Work out the finished part from the listing and answer in its coordinate system (mm). Round coordinates to 2 decimals unless told otherwise and drop trailing zeros. Write each loop counter-clockwise with the first axis right and the second up, starting at its lowest first coordinate (ties: lowest second). Pieces come first, ordered by that corner, then holes. Notation, with made-up numbers: M -7.5,55.25 L 7.5,55.25 A20 ccw 7.5,90.25 Z; hole C 79.25,23.5 d2. An arc over 180 degrees is marked long. Answer in a Markdown table with one row per item.
```python
from build123d import *

# Parameters (mm, degrees)
BOSS_EXTRUDE3_DEPTH     = 5
SKETCH6_R               = 9
CUT_EXTRUDE3_DEPTH      = 4
BOSS_EXTRUDE4_START     = -1
BOSS_EXTRUDE4_OUTLINE_R = 7.6
BOSS_EXTRUDE4_DEPTH     = 1
BOSS_EXTRUDE5_START     = -4
BOSS_EXTRUDE5_OUTLINE_R = 9
BOSS_EXTRUDE5_DEPTH     = 4
BOSS_EXTRUDE6_START     = -1
BOSS_EXTRUDE6_OUTLINE_R = 7.6
BOSS_EXTRUDE6_DEPTH     = 1
CUT_EXTRUDE8_DEPTH      = 20
BOSS_EXTRUDE8_DEPTH     = 5
BOSS_EXTRUDE9_DEPTH     = 5
CUT_EXTRUDE10_DEPTH     = 10


# Read off the part's stored shape, not the designer's step: Boss-Extrude4, Boss-Extrude5, Boss-Extrude6
with BuildPart() as part:
    # Sketch5 → Boss-Extrude3 (new body)
    with BuildSketch(Plane.XY):
        with BuildLine():
            Line((0, 11.5), (120, 11.5))
            ThreePointArc((120, 11.5), (131.5, 0), (120, -11.5))
            Line((120, -11.5), (0, -11.5))
            ThreePointArc((0, -11.5), (-11.5, 0), (0, 11.5))
        make_face()
    extrude(amount=BOSS_EXTRUDE3_DEPTH)

    # Sketch6 → Cut-Extrude3 (cut)
    with BuildSketch(Plane(origin=(0, 0, 0), x_dir=(-1, 0, 0), z_dir=(0, 0, -1))):
        Circle(SKETCH6_R)
    extrude(amount=-CUT_EXTRUDE3_DEPTH, mode=Mode.SUBTRACT)

    # Boss-Extrude4 outline → Boss-Extrude4 (cut)
    with BuildSketch(Plane(origin=(0, 0, 4), x_dir=(-1, 0, 0), z_dir=(0, 0, -1)).offset(BOSS_EXTRUDE4_START)):
        Circle(BOSS_EXTRUDE4_OUTLINE_R)
    extrude(amount=BOSS_EXTRUDE4_DEPTH, mode=Mode.SUBTRACT)

    # Boss-Extrude5 outline → Boss-Extrude5 (cut)
    with BuildSketch(Plane(origin=(0, 0, 0), x_dir=(-1, 0, 0), z_dir=(0, 0, -1)).offset(BOSS_EXTRUDE5_START)):
        with Locations((-120, 0)):
            Circle(BOSS_EXTRUDE5_OUTLINE_R)
    extrude(amount=BOSS_EXTRUDE5_DEPTH, mode=Mode.SUBTRACT)

    # Boss-Extrude6 outline → Boss-Extrude6 (cut)
    with BuildSketch(Plane(origin=(0, 0, 4), x_dir=(-1, 0, 0), z_dir=(0, 0, -1)).offset(BOSS_EXTRUDE6_START)):
        with Locations((-120, 0)):
            Circle(BOSS_EXTRUDE6_OUTLINE_R)
    extrude(amount=BOSS_EXTRUDE6_DEPTH, mode=Mode.SUBTRACT)

    # Sketch12 → Cut-Extrude8 (cut)
    with BuildSketch(Plane.XY.offset(5)):
        with BuildLine():
            Line((16, 7.6), (104, 7.6))
            ThreePointArc((104, 7.6), (106.828427125, 6.428427125), (108, 3.6))
            Line((108, 3.6), (108, -3.748914736))
            ThreePointArc((108, -3.748914736), (106.828427125, -6.577341861), (104, -7.748914736))
            Line((104, -7.748914736), (16, -7.748914736))
            ThreePointArc((16, -7.748914736), (13.171572875, -6.577341861), (12, -3.748914736))
            Line((12, -3.748914736), (12, 3.6))
            ThreePointArc((12, 3.6), (13.171572875, 6.428427125), (16, 7.6))
        make_face()
    extrude(amount=-CUT_EXTRUDE8_DEPTH, mode=Mode.SUBTRACT)

    # Sketch12<10> → Boss-Extrude8 (add)
    with BuildSketch(Plane.XY.offset(5)):
        Polygon((38, -7.748914736), (21, 7.6), (16, 7.6), (33, -7.748914736), align=None)
        Polygon((60, 7.6), (55, 7.6), (38, -7.748914736), (43, -7.748914736), align=None)
        Polygon((65, 7.6), (60, 7.6), (77, -7.748914736), (82, -7.748914736), align=None)
        Polygon((104, 7.6), (99, 7.6), (82, -7.748914736), (87, -7.748914736), align=None)
    extrude(amount=-BOSS_EXTRUDE8_DEPTH)

    # Sketch12<11> → Boss-Extrude9 (add)
    with BuildSketch(Plane.XY.offset(5)):
        with BuildLine():
            ThreePointArc((108, 3.6), (106.828427125, 6.428427125), (104, 7.6))
            Line((104, 7.6), (87, -7.748914736))
            Line((87, -7.748914736), (104, -7.748914736))
            ThreePointArc((104, -7.748914736), (106.828427125, -6.577341861), (108, -3.748914736))
            Line((108, -3.748914736), (108, 3.6))
        make_face()
    extrude(amount=-BOSS_EXTRUDE9_DEPTH)

    # Sketch12<14> → Cut-Extrude10 (cut)
    with BuildSketch(Plane.XY.offset(5)):
        with BuildLine():
            ThreePointArc((108, 3.6), (106.828427125, 6.428427125), (104, 7.6))
            Line((104, 7.6), (87, -7.748914736))
            Line((87, -7.748914736), (104, -7.748914736))
            ThreePointArc((104, -7.748914736), (106.828427125, -6.577341861), (108, -3.748914736))
            Line((108, -3.748914736), (108, 3.6))
        make_face()
    extrude(amount=-CUT_EXTRUDE10_DEPTH, mode=Mode.SUBTRACT)


solid = part.part
```
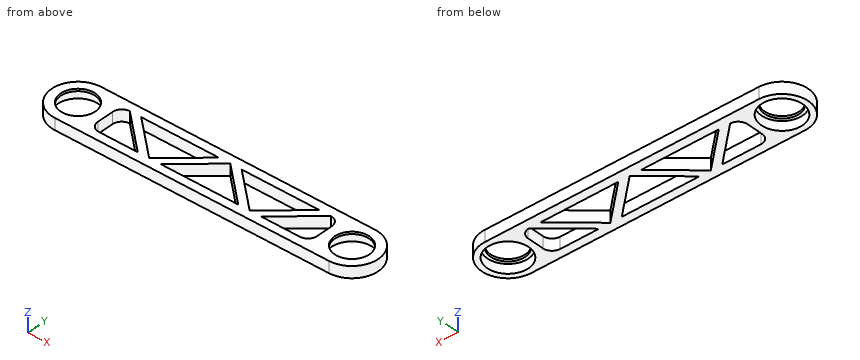
1. Given pin 1 (2 mm diameter, centred on y = -2, z = 2.5, fed in from +X), flat-ended and moving along its own axis, determine where the tip first touches the part or whether it passes through.
Calculated:
| item | result |
|---|---|
| pin 1 | stops at x = 131.46 |
2. Consider line 1 along Y through (x, z) = (49, 2.65); line 2 along Y through (x, z) = (68.5, 0.65); line 3 along Y through (x, z) = (0, 4.5). Determine where each line is inside the solid, lowest interval first. Write a range as from..to.
Calculated:
| item | result |
|---|---|
| line 1 | y = -11.5..-7.75, -2.33..2.18, 7.6..11.5 |
| line 2 | y = -11.5..-7.75, -0.07..4.44, 7.6..11.5 |
| line 3 | y = -11.5..-7.6, 7.6..11.5 |
3. The part is cut by section C-C (y = 5.75). Count the separate pieces of the cut face and the enclosed holes in it, plus the area to 3 significant figures.
Calculated:
| item | result |
|---|---|
| separate pieces | 8 |
| enclosed holes | 0 |
| area | 195 mm² |
4. The part is cut by section A-A (z = 2.25). Determine the outline of the cut face in (x, y).
Calculated:
| item | result |
|---|---|
| outline | M 0,-11.5 L 120,-11.5 A11.5 ccw 120,11.5 L 0,11.5 A11.5 ccw Z; hole C 0,0 d18; hole M 12,-3.75 A4 ccw 16,-7.75 L 33,-7.75 L 16,7.6 A4 ccw 12,3.6 Z; hole M 21,7.6 L 38,-7.75 L 55,7.6 Z; hole M 43,-7.75 L 77,-7.75 L 60,7.6 Z; hole M 65,7.6 L 82,-7.75 L 99,7.6 Z; hole M 87,-7.75 L 104,-7.75 A4 ccw 108,-3.75 L 108,3.6 A4 ccw 104,7.6 Z; hole C 120,0 d18 |
5. The part is cut by section B-B (x = 69.5). Determine the outline of the cut face in (y, z), plus the area to 3 significant figures.
Calculated:
| item | result |
|---|---|
| outline | M -11.5,0 L -7.75,0 L -7.75,5 L -11.5,5 Z; M -0.98,0 L 3.54,0 L 3.54,5 L -0.98,5 Z; M 7.6,0 L 11.5,0 L 11.5,5 L 7.6,5 Z |
| area | 60.8 mm² |
